Verification items for this drawing (mm, ordinates from the low corner). A direction names the side the tool comes from. Round coordinates to 2 decimals unless told otherwise and drop trailing zeros. Order: outer loops, then holes, each group sorted by start corner. A loop starts at its lowest first (then second) coordinate and runs counter-clockwise, first axis right, second up. Notation, with made-up numbers: (-18, -14.5) -> (35, -14.5) arc R33 cw to (35, 16.5) -> close; hole circle Ø5 at (53, 81). An arc over 180 degrees is marked (long way). Answer in a Markdown table with one row per item. Add a question column.
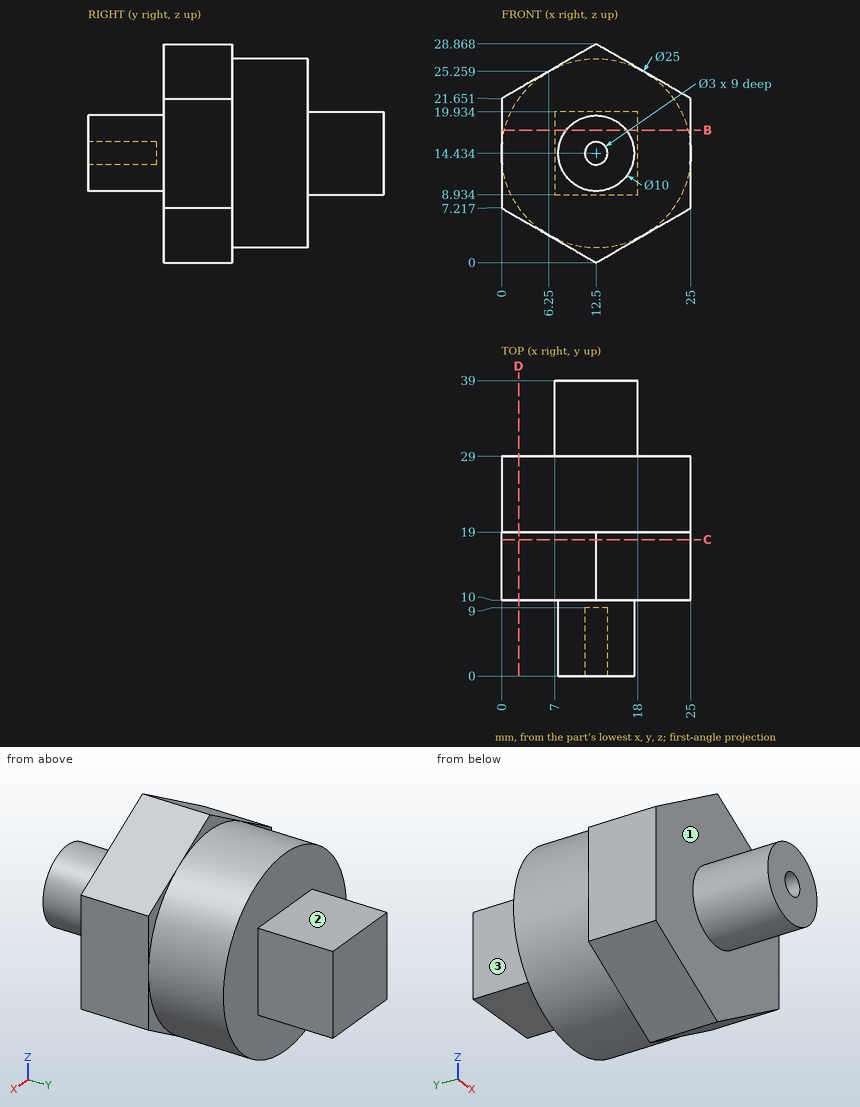
1) Depth check by flat-ended pin: P1, Ø8, axis at x = 10.5, y = 5.5, coming from the +Z side; P2, Ø5, axis at x = 7.5, y = 10, coming from the +Z side (1 decimal); P3, Ø1.5, axis at x = 12.5, z = 14, coming from the -Y side. Enter the tip coordinate at first touch or a pass-through.
2) Thickness scan on L1, parallel to Z at x = 12.5, y = 6.75; L2, parallel to Y at x = 7.75, z = 7; L3, parallel to Y at x = 7.5, z = 18.25. Record the ranges inside material, lowest first. Write a range as [from, to].
3) Cross-section at D-D, the plane x = 2.25. Record the boundary of the cut face in (y, z), and give its area (3 significant figures).
4) Cross-section at B-B, the plane z = 17.5. Record the boundary of the cut face in (x, y).
5) Tool access check on the marked faces 1, 2 and 3. Record the directions out of +Z, -Z, +X, -X, +Y, -Y that give a thin tool (end or side, any length) a straight path to the whole face; none if there is none.
6) Cross-section at C-C, the plane y = 18. Record the boundary of the cut face in (x, z).
Results below:
| question | item | result |
|---|---|---|
| 1 | P1 | z = 19.43 |
| 1 | P2 | z = 27.4 |
| 1 | P3 | y = 9 |
| 2 | L1 | [9.43, 12.93], [15.93, 19.43] |
| 2 | L2 | [10, 29] |
| 2 | L3 | [10, 39] |
| 3 | outline | (10, 5.92) -> (19, 5.92) -> (19, 7.28) -> (29, 7.28) -> (29, 21.59) -> (19, 21.59) -> (19, 22.95) -> (10, 22.95) -> close |
| 3 | area | 296 mm² |
| 4 | outline | (0, 10) -> (8.55, 10) -> (8.55, 0) -> (16.45, 0) -> (16.45, 10) -> (25, 10) -> (25, 19) -> (24.62, 19) -> (24.62, 29) -> (18, 29) -> (18, 39) -> (7, 39) -> (7, 29) -> (0.38, 29) -> (0.38, 19) -> (0, 19) -> close |
| 5 | face 1 | -Y |
| 5 | face 2 | +Z, +X, -X, +Y |
| 5 | face 3 | +Z, -Z, -X, +Y |
| 6 | outline | (0, 7.22) -> (12.5, 0) -> (25, 7.22) -> (25, 21.65) -> (12.5, 28.87) -> (0, 21.65) -> close |
